Model file for the job. Use its own axes, mm. A direction names the side the tool comes from. Give positions to 0.01 mm unless a question says otherwise; leave off trailing zeros. Write each loop counter-clockwise with the first axis right and the second up, starting at its lowest first coordinate (ties: lowest second). Pieces come first, ordered by that corner, then holes. Notation, with made-up numbers: (71.5, -10.75) - (116.5, -10.75) arc R11 ccw to (116.5, -1.75) - close; hole circle Ø10 at (-37, 51). An arc over 180 degrees is marked (long way). One line per item, written item: value. Start each with the question number.
(1) Drop a flat-ended pin along its axis: P1, Ø5.5, axis at y = -3.81, z = 454.914, coming from the +X side. Give the stop position or say it passes through.
(2) Probe L1, parallel to X at y = 8, z = 279 (3 decimals); L2, parallel to Y at x = 11, z = 405.75. List the from-to ranges inside material, lowest first.
(3) 3-axis set-ups, long thin cutter, end or side, ignore diameter. For faces 1 (the face through (1.43, 11.09, 373.98)), 2 (the face through (9.525, 0, 282)): which of +Z, -Z, +X, -X, +Y, -Y reach the whole face in a straight line?
(4) Mould opens along Z. For faces 3 (the face through (11, 0, 571.5)), 4 (the face through (-12.7, 0, 282)), 5 (the face through (0.21, -11.13, 326.13)) say: pulls with the +Z half, pulls with the -Z half, needs draft (parallel to the pull), parting line crosses it, or undercut.
(5) Cut at A-A, the plane z = 232.5. List the corners of the cut face in (x, y) (3 decimals).
from build123d import *

# Parameters (mm, degrees)
SKETCH1_W                    = 25.4
SKETCH1_H                    = 25.4
SKETCH1_W_2                  = 19.05
SKETCH1_H_2                  = 19.05
EXTRUDE_THIN1_DEPTH          = 571.5
F_8_CLEARANCE_HOLE1_D        = 4.4958
F_8_32_TAPPED_HOLE1_D        = 3.4544
F_8_32_TAPPED_HOLE1_DEPTH    = 12.2936
F_8_32_TAPPED_HOLE1_TIP      = 1.037806461
F_3_8_0_375_DIAMETER_HOLE2_D = 9.525
F_3_8_0_375_DIAMETER_HOLE3_D = 9.525


with BuildPart() as part:
    # Sketch1 → Extrude-Thin1 (new body)
    with BuildSketch(Plane.XY):
        Rectangle(SKETCH1_W, SKETCH1_H)
        Rectangle(SKETCH1_W_2, SKETCH1_H_2, mode=Mode.SUBTRACT)
    extrude(amount=EXTRUDE_THIN1_DEPTH)

    # #8 Clearance Hole1 (through all)
    with Locations(Plane(origin=(0, 12.7, 565.15), x_dir=(0, 0, 1), z_dir=(0, 1, 0))):
        with Locations((0, 0), (-558.8, 0), (-533.4, 0), (-508, 0), (-25.4, 0), (-50.8, 0)):
            Hole(F_8_CLEARANCE_HOLE1_D / 2)

    # #8-32 Tapped Hole1
    with Locations(Plane(origin=(12.7, -82.55, 285.75), x_dir=(0, 0, -1), z_dir=(1, 0, 0))):
        with Locations((-240, 82.55), (-120, 82.55), (-60, 82.55), (0, 82.55), (60, 82.55), (120, 82.55), (240, 82.55)):
            Hole(F_8_32_TAPPED_HOLE1_D / 2, depth=F_8_32_TAPPED_HOLE1_DEPTH)
            with Locations((0, 0, -(F_8_32_TAPPED_HOLE1_DEPTH + F_8_32_TAPPED_HOLE1_TIP / 2))):  # 118° drill point
                Cone(0, F_8_32_TAPPED_HOLE1_D / 2, F_8_32_TAPPED_HOLE1_TIP, mode=Mode.SUBTRACT)

    # 3/8 (0.375) Diameter Hole2 (through all)
    with Locations(Plane(origin=(-12.7, -82.55, 285.75), x_dir=(0, 0, -1), z_dir=(-1, 0, 0))):
        with Locations((-181.864, -86.995), (-169.164, -78.74), (169.164, -78.74), (181.864, -86.995), (181.864, -57.15), (-181.864, -57.15)):
            Hole(F_3_8_0_375_DIAMETER_HOLE2_D / 2)

    # 3/8 (0.375) Diameter Hole3 (through all)
    with Locations(Plane(origin=(-346.075, 12.7, 285.75), x_dir=(0, 0, 1), z_dir=(0, 1, 0))):
        with Locations((-92.7735, 346.075), (-35.6235, 346.075), (35.6235, 346.075), (92.7735, 346.075), (-19.05, -346.775), (53.975, -346.775), (127, -346.775), (-381, -114.3), (-381, -130.175), (-381, -146.05), (-381, 114.3), (-381, 98.425), (-381, 82.55)):
            Hole(F_3_8_0_375_DIAMETER_HOLE3_D / 2)


solid = part.part
Answers follow:
1. P1: passes through
2. L1: x = -12.7 to -9.525, 9.525 to 12.7
2. L2: y = -12.7 to -1.73, 1.73 to 12.7
3. face 1: +Y, -Y
3. face 2: +Z, -Z
4. face 3: pulls with the +Z half
4. face 4: needs draft
4. face 5: undercut
5. outline: (-12.7, -12.7) - (12.7, -12.7) - (12.7, 12.7) - (-12.7, 12.7) - close; hole (-9.525, -9.525) - (9.525, -9.525) - (9.525, 9.525) - (-9.525, 9.525) - close
